```python
from build123d import *

# Parameters (mm, degrees)
F1_DEPTH = 1


with BuildPart() as f1:
    # F0 (on Front) → F1 (new body)
    with BuildSketch(Plane.XZ):
        with BuildLine():
            Line((10, 52), (-10, 52))
            ThreePointArc((-10, 52), (-19.134172, 46.193977), (-29.698485, 43.84062))
            Line((-29.698485, 43.84062), (-43.84062, 29.698485))
            ThreePointArc((-43.84062, 29.698485), (-46.193977, 19.134172), (-52, 10))
            Line((-52, 10), (-52, -10))
            ThreePointArc((-52, -10), (-46.193977, -19.134172), (-43.84062, -29.698485))
            Line((-43.84062, -29.698485), (-29.698485, -43.84062))
            ThreePointArc((-29.698485, -43.84062), (-19.134172, -46.193977), (-10, -52))
            Line((-10, -52), (10, -52))
            ThreePointArc((10, -52), (19.134172, -46.193977), (29.698485, -43.84062))
            Line((29.698485, -43.84062), (43.84062, -29.698485))
            ThreePointArc((43.84062, -29.698485), (46.193977, -19.134172), (52, -10))
            Line((52, -10), (52, 10))
            ThreePointArc((52, 10), (46.193977, 19.134172), (43.84062, 29.698485))
            Line((43.84062, 29.698485), (29.698485, 43.84062))
            ThreePointArc((29.698485, 43.84062), (19.134172, 46.193977), (10, 52))
        make_face()
    extrude(amount=F1_DEPTH)


solid = f1.part
```
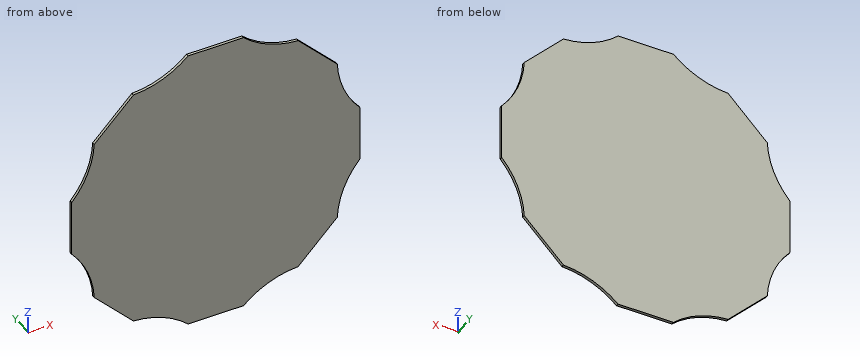
Geometry: final body of the model. Coordinates: model frame, mm. Round coordinates to 2 decimals unless told otherwise and drop trailing zeros. Order: outer loops, then holes, each group sorted by start corner. A loop starts at its lowest first (then second) coordinate and runs counter-clockwise, first axis right, second up. Notation, with made-up numbers: M 53,74.25 L 61,74.25 A20 cw 61,109.25 Z; hole C 60,43.25 d5. An arc over 180 degrees is marked long. Use one line per item in the form item = value. Start each with the question number.
Q1. Cut plane C-C (x = 16). Return loops of the section in (y, z).
Q2. Cut plane A-A (y = -0.65). Return loops of the section in (x, z).
Q3. Material intervals for line 1 (X direction, y = -0.9, z = 28); line 2 (X direction, y = -0.7, z = -31.5); line 3 (Z direction, x = 42, y = -0.05), sorted ascending. Write a range as [from, to].
Q4. Cut plane B-B (z = -31.5). Return loops of the section in (x, y), and give its area (3 significant figures).
Geometry results:
q1.outline = M -1,-47.7 L 0,-47.7 L 0,47.7 L -1,47.7 Z
q2.outline = M -52,-10 A31.35 cw -43.84,-29.7 L -29.7,-43.84 A31.35 cw -10,-52 L 10,-52 A31.35 cw 29.7,-43.84 L 43.84,-29.7 A31.35 cw 52,-10 L 52,10 A31.35 cw 43.84,29.7 L 29.7,43.84 A31.35 cw 10,52 L -10,52 A31.35 cw -29.7,43.84 L -43.84,29.7 A31.35 cw -52,10 Z
q3.line_1 = [-43.96, 43.96]
q3.line_2 = [-42.04, 42.04]
q3.line_3 = [-31.54, 31.54]
q4.outline = M -42.04,-1 L 42.04,-1 L 42.04,0 L -42.04,0 Z
q4.area = 84.1 mm^2
